```python
from build123d import *


with BuildPart() as part:
    # Sketch1 → Revolve1 (revolve)
    with BuildSketch(Plane.XY):
        with BuildLine():
            Line((2.54, 7.62), (-2.54, 7.62))
            Line((-2.54, 7.62), (-2.54, 5.953125))
            Line((-2.54, 5.953125), (-2.209706481, 5.953125))
            ThreePointArc((-2.209706481, 5.953125), (0, 6.35), (2.209706481, 5.953125))
            Line((2.209706481, 5.953125), (2.54, 5.953125))
            Line((2.54, 5.953125), (2.54, 7.62))
        make_face()
    revolve(axis=Axis((-10.16, 0, 0), (1, 0, 0)))

    # Sketch2 → Revolve2 (revolve)
    with BuildSketch(Plane(origin=(0, 0, 0), x_dir=(0, 0, -1), z_dir=(1, 0, 0))):
        with BuildLine():
            Line((1.27, -7.513421325), (1.27, -33.02))
            Line((1.27, -33.02), (0, -33.02))
            Line((0, -33.02), (0, -7.62))
            ThreePointArc((0, -7.62), (0.637232103, -7.593308584), (1.27, -7.513421325))
        make_face()
    revolve(axis=Axis((0, -33.02, 0), (0, 1, 0)))


solid = part.part
```
Here's how the part is built. I have some questions about the finished solid (model axes, mm). Give positions to 0.01 mm unless a question says otherwise; leave off trailing zeros. Write each loop counter-clockwise with the first axis right and the second up, starting at its lowest first coordinate (ties: lowest second). Pieces come first, ordered by that corner, then holes. Notation, with made-up numbers: (22.25, -28.75) -> (52.25, -28.75) arc R26 ccw to (52.25, 7.25) -> close; hole circle Ø9 at (58.25, 57.25). An arc over 180 degrees is marked (long way). Use one line per item in the form item = value.
1) Suppose I cut it at D-D (y = -20). Please give me the cut outline in (x, z), and give its area (3 significant figures).
Verdict:
outline = circle Ø2.54 at (0, 0)
area = 5.07 mm2
2) If I drill on L1, parallel to Z at x = 2.35, y = 0; L2, parallel to Y at x = 1.4, z = -0.5; L3, parallel to Y at x = -1.45, z = 4, over which ranges is the centre line in solid material (lowest first)? Write a range as [from, to].
Verdict:
L1 = [-7.62, -5.95], [5.95, 7.62]
L2 = [-7.6, -6.17], [6.17, 7.6]
L3 = [-6.49, -4.71], [4.71, 6.49]
3) I'm going to push flat-ended pins straight in: pin 1 (3 mm diameter, centred on x = 1.5, y = -25, fed in from -Z); pin 2 (6 mm diameter, centred on y = -7.5, z = -2.5, fed in from +X). Where does each tip first touch, or does it pass through?
Verdict:
pin_1 = -1.27
pin_2 = 2.54
4) Suppose I cut it at C-C (z = 5.5). Please give me the cut outline in (x, y).
Verdict:
outline = (-2.54, -5.27) -> (2.54, -5.27) -> (2.54, -2.28) -> (2.21, -2.28) arc R3.17 cw to (-2.21, -2.28) -> (-2.54, -2.28) -> close; (-2.54, 2.28) -> (-2.21, 2.28) arc R3.17 cw to (2.21, 2.28) -> (2.54, 2.28) -> (2.54, 5.27) -> (-2.54, 5.27) -> close
5) Suppose I cut it at A-A (y = 0). Please give me the cut outline in (x, z).
Verdict:
outline = (-2.54, -7.62) -> (2.54, -7.62) -> (2.54, -5.95) -> (2.21, -5.95) arc R6.35 cw to (-2.21, -5.95) -> (-2.54, -5.95) -> close; (-2.54, 5.95) -> (-2.21, 5.95) arc R6.35 cw to (2.21, 5.95) -> (2.54, 5.95) -> (2.54, 7.62) -> (-2.54, 7.62) -> close
6) We'd pull the mould along Z, two halves only. Please class faces 1 (the face through (-2.54, -5, -4)), 2 (the face through (-1.26, -20.45, 0.17)), 3 (the face through (-2.373, -4.724, -3.622)): +Z half, -Z half, draft (parallel to the pull), parting line (faces both ways), or undercut.
Verdict:
face_1 = draft
face_2 = parting line
face_3 = undercut
7) Suppose I cut it at B-B (x = 0). Please give me the cut outline in (y, z).
Verdict:
outline = (-33.02, -1.27) -> (-7.51, -1.27) arc R7.62 ccw (long way) to (-7.51, 1.27) -> (-33.02, 1.27) -> close; hole circle Ø12.7 at (0, 0)
